```python
from build123d import *

# Parameters (mm, degrees)
F0_R     = 28.5
F1_DEPTH = 11
F3_DEPTH = 1
F4_R     = 2.75
F5_DEPTH = 6.4
F6_DEPTH = 8
F7_R     = 28.5
F7_R_2   = 27
F8_DEPTH = 4
F10_SIZE = 2


# Not quite as in the source:
# - a fillet or chamfer that OpenCascade refuses, or shapes differently, is made with other operations: its cross-section is extruded or revolved along the edge and cut away or added


with BuildPart() as f1:
    # F0 (on Top) → F1 (new body)
    with BuildSketch(Plane.XY):
        Circle(F0_R)
    extrude(amount=F1_DEPTH)

    # F2 (on face) → F3 (cut)
    with BuildSketch(Plane(origin=(0, 0, 0), x_dir=(1, 0, 0), z_dir=(0, 0, -1))):
        Polygon((10.68097998, 18.5), (-10.68097998, 18.5), (-21.36195996, 0), (-10.68097998, -18.5), (10.68097998, -18.5), (21.36195996, 0), align=None)
    extrude(amount=-F3_DEPTH, mode=Mode.SUBTRACT)

    # F4 (on face) → F5 (cut)
    with BuildSketch(Plane.XY.offset(11)):
        Circle(F4_R)
    extrude(amount=-F5_DEPTH, mode=Mode.SUBTRACT)

    # F6 (add): a face of the model
    f6_faces = [f1.faces().sort_by_distance(p)[0] for p in [
        (-27.6938982694, 0, 0),
    ]]
    extrude(f6_faces, amount=F6_DEPTH)

    # F7 (on face) → F8 (join)
    with BuildSketch(Plane(origin=(0, 0, -8), x_dir=(1, 0, 0), z_dir=(0, 0, -1))):
        Circle(F7_R)
        Circle(F7_R_2, mode=Mode.SUBTRACT)
    extrude(amount=F8_DEPTH)

    # F9: chamfer of 2 on 1 edges, made by hand

    # F9_s1 → F9_t2 (revolve, cut)
    with BuildSketch(Plane.XZ):
        Polygon((29, -12), (27, -10), (27, -12), align=None)
    revolve(axis=Axis((0, 0, -12), (0, 0, -1)), mode=Mode.SUBTRACT)

    # F10
    f10_edges = [f1.edges().sort_by_distance(p)[0] for p in [
        (0, -18.5, -8),
        (16.02147, -9.25, -8),
        (16.02147, 9.25, -8),
        (0, 18.5, -8),
        (-16.02147, 9.25, -8),
        (-16.02147, -9.25, -8),
    ]]
    chamfer(f10_edges, length=F10_SIZE)


solid = f1.part
```
Geometry check sheet. Reference: the model listing, model coordinates, mm. A direction names the side the tool comes from. Round coordinates to 2 decimals unless told otherwise and drop trailing zeros. Order: outer loops, then holes, each group sorted by start corner. A loop starts at its lowest first (then second) coordinate and runs counter-clockwise, first axis right, second up. Notation, with made-up numbers: (-27.5, -20.75) - (-16.5, -20.75) arc R30 ccw to (-16.5, 4.25) - close; hole circle Ø7 at (-12, -8.75). An arc over 180 degrees is marked (long way). Use a Markdown table: item, result. Add a question column.
1) Section check D-D (z = 9.5). Record the cut outline in (x, y).
2) Gauge pin test, flat ends, axial feed: P1, Ø1, axis at y = -14, z = -7.5, coming from the +X side; P2, Ø7.5, axis at x = -0.5, z = -1, coming from the +Y side; P3, Ø3, axis at y = 20, z = 7, coming from the -X side. Record the tip position at first contact, or that the pin passes through.
3) Section check C-C (z = 2.75). Record the cut outline in (x, y).
4) Set-up check for faces 3 (the flat face through (0, 18.5, -2)), 4 (the flat face through (0, 0, 4.6)): record each of +Z, -Z, +X, -X, +Y, -Y from which the full face is reachable in a straight line by a thin tool's end or side.
5) Section check A-A (x = 0). Record the cut outline in (y, z), then the cut area to 3 significant figures.
6) Thickness scan on line 1 along Y through (x, z) = (0, -8.55); line 2 along Y through (x, z) = (-0.5, -5.5); line 3 along Z through (x, y) = (-6.5, -4). Record the ranges inside material, lowest first.
7) Mould release check, pull along Y, two halves, no side actions. Record for faces 1 (the flat face through (0, -6, 11)), 2 (the cylindrical face through (-0.596, -2.685, 7.845)): released by +Y, released by -Y, zero draft, split by the parting line, or undercut.
8) Section check B-B (z = -0.5). Record the cut outline in (x, y), then the cut area to 3 significant figures.
Established:
| question | item | result |
|---|---|---|
| 1 | outline | circle Ø57 at (0, 0); hole circle Ø5.5 at (0, 0) |
| 2 | P1 | x = 25.1 |
| 2 | P2 | y = 28.5 |
| 2 | P3 | x = -21.68 |
| 3 | outline | circle Ø57 at (0, 0) |
| 4 | face 3 | -Z |
| 4 | face 4 | +Z |
| 5 | outline | (-28.5, -11.5) - (-27, -10) - (-27, -8) - (-20.5, -8) - (-18.5, -6) - (-18.5, 1) - (18.5, 1) - (18.5, -6) - (20.5, -8) - (27, -8) - (27, -10) - (28.5, -11.5) - (28.5, 11) - (2.75, 11) - (2.75, 4.6) - (-2.75, 4.6) - (-2.75, 11) - (-28.5, 11) - close |
| 5 | area | 719 mm2 |
| 6 | line 1 | -28.5 to -27, 27 to 28.5 |
| 6 | line 2 | -28.5 to -18.5, 18.5 to 28.5 |
| 6 | line 3 | 1 to 11 |
| 7 | face 1 | zero draft |
| 7 | face 2 | undercut |
| 8 | outline | circle Ø57 at (0, 0); hole (-21.36, 0) - (-10.68, -18.5) - (10.68, -18.5) - (21.36, 0) - (10.68, 18.5) - (-10.68, 18.5) - close |
| 8 | area | 1,370 mm2 |
